from build123d import *

# Parameters (mm, degrees)
F0_W          = 5.842
F0_H          = 12.7
F0_R          = 3.175
F2_DEPTH      = 3.175
F3_R          = 1.524
F4_DEPTH      = 7.62
F4_DEPTH_BACK = 1.27
F5_DEPTH      = 56.134
F8_DEPTH      = 17.78
F9_DEPTH      = 10.414
F10_R         = 1.27


with BuildPart() as f1:
    # F0 (on Front) → F1 (revolve)
    with BuildSketch(Plane.XZ):
        Polygon((5.842, 12.7), (5.842, 0), (66.294, 0), (66.294, 12.7), (56.134, 12.7), (56.134, 10.16), (10.16, 10.16), (10.16, 12.7), align=None)
        with Locations((2.921, 6.35)):
            Rectangle(F0_W, F0_H)
    revolve(axis=Axis((33.147, 0, 0), (-1, 0, 0)))

    # F0 (on Front) → F2 (join, symmetric)
    with BuildSketch(Plane.XZ):
        with BuildLine():
            ThreePointArc((-8.1826630726, -5.5069827884), (-3.1957909266, -4.5493385486), (-0.9398, 0))
            ThreePointArc((-0.9398, 0), (-4.5919612295, 5.3297205562), (-10.8806298187, 3.8475430269))
            ThreePointArc((-10.8806298187, 3.8475430269), (-12.1459778134, -1.5837270034), (-8.1826630726, -5.5069827884))
        make_face()
        with Locations((-6.6548, 0)):
            Circle(F0_R, mode=Mode.SUBTRACT)
        with BuildLine():
            Line((-0.9398, 0), (0, 0))
            Line((0, 0), (0, 12.7))
            Line((0, 12.7), (5.842, 12.7))
            Line((5.842, 12.7), (5.842, 15.24))
            Line((5.842, 15.24), (-0.508, 15.24))
            Line((-0.508, 15.24), (-10.8806298187, 3.8475430269))
            ThreePointArc((-10.8806298187, 3.8475430269), (-4.5919612295, 5.3297205562), (-0.9398, 0))
        make_face()
        with Locations((2.921, 6.35)):
            Rectangle(F0_W, F0_H)
        with BuildLine():
            Line((5.842, 0), (0, 0))
            Line((0, 0), (-0.9398, 0))
            ThreePointArc((-0.9398, 0), (-3.1957909266, -4.5493385486), (-8.1826630726, -5.5069827884))
            Line((-8.1826630726, -5.5069827884), (5.842, -9.398))
            Line((5.842, -9.398), (5.842, 0))
        make_face()
    extrude(amount=F2_DEPTH, both=True)

    # F3 (on face) → F4 (join, two sides)
    with BuildSketch(Plane.YZ.offset(66.294)) as f4_sk:
        with BuildLine():
            ThreePointArc((-5.08, 11.6397422652), (0, 12.7), (5.08, 11.6397422652))
            Line((5.08, 11.6397422652), (5.08, 15.24))
            Line((5.08, 15.24), (-5.08, 15.24))
            Line((-5.08, 15.24), (-5.08, 11.6397422652))
        make_face()
        with BuildLine():
            ThreePointArc((-5.08, 0), (0, -5.08), (5.08, 0))
            ThreePointArc((5.08, 0), (0, 5.08), (-5.08, 0))
        make_face()
        Circle(F3_R, mode=Mode.SUBTRACT)
        with BuildLine():
            ThreePointArc((-5.08, 0), (0, 5.08), (5.08, 0))
            Line((5.08, 0), (5.08, 11.6397422652))
            ThreePointArc((5.08, 11.6397422652), (0, 12.7), (-5.08, 11.6397422652))
            Line((-5.08, 11.6397422652), (-5.08, 0))
        make_face()
    extrude(amount=F4_DEPTH)
    extrude(f4_sk.sketch, amount=-F4_DEPTH_BACK)

    # F5 (cut, through all): a face of the model
    f5_faces = [f1.faces().sort_by_distance(p)[0] for p in [
        (66.294, 0, 0),
    ]]
    extrude(f5_faces, amount=-F5_DEPTH, mode=Mode.SUBTRACT)

    # F6 (on face) → F8 (cut)
    with BuildSketch(Plane.XY.offset(15.24)):
        with BuildLine():
            ThreePointArc((2.667, -1.524), (3.7446307345, -1.0776307345), (4.191, 0))
            ThreePointArc((4.191, 0), (3.7446307345, 1.0776307345), (2.667, 1.524))
            ThreePointArc((2.667, 1.524), (1.143, 0), (2.667, -1.524))
        make_face()
    extrude(amount=-F8_DEPTH, mode=Mode.SUBTRACT)

    # F7 (on face) → F9 (cut)
    with BuildSketch(Plane.XY.offset(15.24)):
        with BuildLine():
            ThreePointArc((70.993, 0), (70.5466307345, 1.0776307345), (69.469, 1.524))
            ThreePointArc((69.469, 1.524), (67.945, 0), (69.469, -1.524))
            ThreePointArc((69.469, -1.524), (70.5466307345, -1.0776307345), (70.993, 0))
        make_face()
    extrude(amount=-F9_DEPTH, mode=Mode.SUBTRACT)

    # F10
    f10_edges = [f1.edges().sort_by_distance(p)[0] for p in [
        (56.134, 0, -12.7),
        (66.294, 0, -12.7),
        (10.16, 0, -12.7),
        (0, 0, -12.7),
    ]]
    fillet(f10_edges, radius=F10_R)


solid = f1.part
Check sheet for the modelled part. Datum: model origin and axes. Units: mm. A direction names the side the tool comes from. Round coordinates to 2 decimals unless told otherwise and drop trailing zeros. Order: outer loops, then holes, each group sorted by start corner. A loop starts at its lowest first (then second) coordinate and runs counter-clockwise, first axis right, second up.
(1) Scan lines: probe 1 along X at (y, z) = (5.25, 10); probe 2 along X at (y, z) = (-7, 7); probe 3 along X at (y, z) = (5, 3). Record each from-to range of solid material in increasing order.
(2) Cross-section at B-B, the plane x = 58.5. Enter the section's corners in (y, z), and give its area (3 significant figures).
(3) Cross-section at A-A, the plane x = 31. Enter the section's corners in (y, z).
(4) Access from +Z, -Z, +X, -X, +Y, -Y to the whole of each face (thin tool, end or side, straight path). Record for faces 1 (the cylindrical face through (32.825, 10.074, -1.323)), 2 (the flat face through (-5.622, -0.044, 9.624)), 3 (the flat face through (66.294, 0.2, -5.3)), 4 (the cylindrical face through (-12.168, -0.044, -1.505)), 5 (the flat face through (69, 0, 4.826)).
(5) Draft check along X on faces 6 (the flat face through (-4.149, -0.044, -6.626)), 7 (the flat face through (10.16, -7, 8)), 8 (the cylindrical face through (41.59, -0.2, 1.51)). Enter one of: pulls with the +X half, pulls with the -X half, needs draft (parallel to the pull), parting line crosses it, or undercut.
(6) Go/stop test with flat-tipped pins: P1, Ø5, axis at y = -9.5, z = 12, coming from the +X side; P2, Ø0.9, axis at x = 69.5, y = 0, coming from the +Z side; P3, Ø10, axis at y = -10, z = -5, coming from the -X side; P4, Ø1.8, axis at y = -1.5, z = 12.5, coming from the -X side. Record where each tip stops, or that it passes through.
Check sheet entries:
1. probe 1: x = 0 to 10.16, 56.13 to 66.29
1. probe 2: x = 0 to 66.29
1. probe 3: x = 0 to 73.91
2. outline: circle Ø25.4 at (0, 0); hole circle Ø3.05 at (0, 0)
2. area: 499 mm2
3. outline: circle Ø20.32 at (0, 0); hole circle Ø3.05 at (0, 0)
4. face 1: none
4. face 2: +Z, -X, +Y, -Y
4. face 3: -Z, +X
4. face 4: -X, +Y, -Y
4. face 5: +Z
5. face 6: pulls with the -X half
5. face 7: undercut
5. face 8: needs draft
6. P1: passes through
6. P2: stops at z = 4.83
6. P3: stops at x = 0
6. P4: stops at x = -3.82
